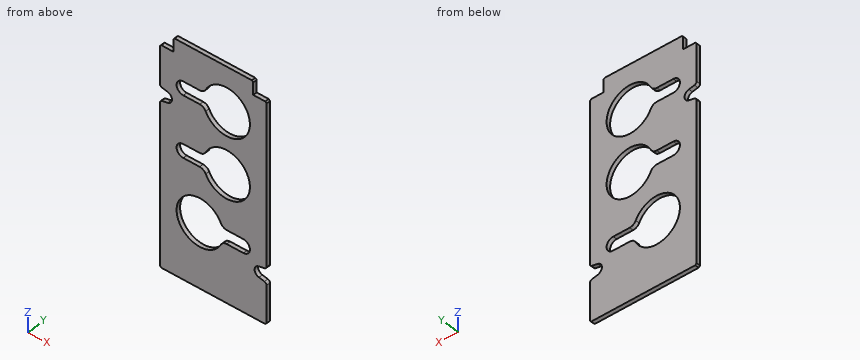
```python
from build123d import *

# Parameters (mm, degrees)
SKETCH226_R     = 17.5
PAD114_DEPTH    = 3
POCKET054_DEPTH = 3.001
FILLET072_R     = 2
CHAMFER079_SIZE = 1
POCKET055_DEPTH = 5
FILLET073_R     = 5


with BuildPart() as part:
    # Sketch226 → Pad114 (new body)
    with BuildSketch(Plane.XZ):
        Polygon((40, 150), (-40, 150), (-40, 310), (-30, 310), (-30, 320), (30, 320), (30, 310), (40, 310), align=None)
        with Locations((10, 287.5)):
            Circle(SKETCH226_R, mode=Mode.SUBTRACT)
        with Locations((10, 242.5)):
            Circle(SKETCH226_R, mode=Mode.SUBTRACT)
        with Locations((-10, 197.5)):
            Circle(SKETCH226_R, mode=Mode.SUBTRACT)
    extrude(amount=-PAD114_DEPTH)

    # Sketch227 → Pocket054 (cut, through all)
    with BuildSketch(Plane.XZ):
        with BuildLine():
            ThreePointArc((-39, 279.898979), (-45, 275), (-39, 270.101021))
            Line((-39, 270.101021), (-34.2, 271.080816))
            ThreePointArc((-34.2, 271.080816), (-31, 275), (-34.2, 278.919184))
            Line((-34.2, 278.919184), (-39, 279.898979))
        make_face()
        with BuildLine():
            ThreePointArc((39, 180.101021), (45, 185), (39, 189.898979))
            Line((39, 189.898979), (34.2, 188.919184))
            ThreePointArc((34.2, 188.919184), (31, 185), (34.2, 181.080816))
            Line((34.2, 181.080816), (39, 180.101021))
        make_face()
    extrude(amount=-POCKET054_DEPTH, mode=Mode.SUBTRACT)

    # Fillet072
    fillet072_edges = [part.edges().sort_by_distance(p)[0] for p in [
        (40, 1.5, 180),
        (40, 1.5, 190),
        (-40, 1.5, 270),
        (-40, 1.5, 280),
    ]]
    fillet(fillet072_edges, radius=FILLET072_R)

    # Chamfer079
    chamfer079_edges = [part.edges().sort_by_distance(p)[0] for p in [
        (-30, 1.5, 320),
        (-40, 1.5, 310),
        (30, 1.5, 320),
        (40, 1.5, 310),
        (-40, 1.5, 150),
        (40, 1.5, 150),
    ]]
    chamfer(chamfer079_edges, length=CHAMFER079_SIZE)

    # Sketch228 → Pocket055 (cut)
    with BuildSketch(Plane.XZ):
        with BuildLine():
            ThreePointArc((10, 282.5), (15, 287.5), (10, 292.5))
            Line((10, 292.5), (-22.5, 292.5))
            ThreePointArc((-22.5, 292.5), (-27.5, 287.5), (-22.5, 282.5))
            Line((-22.5, 282.5), (10, 282.5))
        make_face()
        with BuildLine():
            ThreePointArc((10, 237.5), (15, 242.5), (10, 247.5))
            Line((10, 247.5), (-22.5, 247.5))
            ThreePointArc((-22.5, 247.5), (-27.5, 242.5), (-22.5, 237.5))
            Line((-22.5, 237.5), (10, 237.5))
        make_face()
        with BuildLine():
            ThreePointArc((-10, 202.5), (-15, 197.5), (-10, 192.5))
            Line((-10, 192.5), (22.5, 192.5))
            ThreePointArc((22.5, 192.5), (27.5, 197.5), (22.5, 202.5))
            Line((22.5, 202.5), (-10, 202.5))
        make_face()
    extrude(amount=-POCKET055_DEPTH, mode=Mode.SUBTRACT)

    # Fillet073
    fillet073_edges = [part.edges().sort_by_distance(p)[0] for p in [
        (-6.77051, 1.5, 292.5),
        (-6.77051, 1.5, 282.5),
        (-6.77051, 1.5, 237.5),
        (-6.77051, 1.5, 247.5),
        (6.77051, 1.5, 192.5),
        (6.77051, 1.5, 202.5),
    ]]
    fillet(fillet073_edges, radius=FILLET073_R)


with BuildPart() as part_1:
    # Body098 placement: moved
    add(part.part.moved(Location((0, 75, 0))))


solid = part_1.part
```
Verification items for the finished model (mm, model axes). Give positions to 0.01 mm unless a question says otherwise; leave off trailing zeros. Order: outer loops, then holes, each group sorted by start corner. A loop starts at its lowest first (then second) coordinate and runs counter-clockwise, first axis right, second up. Notation, with made-up numbers: (19, 9.5) -> (61, 9.5) arc R11 ccw to (61, 21.5) -> close; hole circle Ø1 at (12, 77). An arc over 180 degrees is marked (long way). One line per item, written item: value.
(1) Scan lines: line 1 along Z through (x, y) = (-10, 76.2); line 2 along Z through (x, y) = (10, 76.35); line 3 along X through (y, z) = (77.15, 242.5). Record each from-to range of solid material in increasing order. Write a range as [from, to].
Final values:
line 1: [150, 180], [215, 237.5], [247.5, 282.5], [292.5, 320]
line 2: [150, 192.5], [202.5, 225], [260, 270], [305, 320]
line 3: [-40, -27.5], [27.5, 40]
(2) Gauge pin test, flat ends, axial feed: pin 1 (0.9 mm diameter, centred on x = -34, y = 76.5, fed in from +Z); pin 2 (0.9 mm diameter, centred on y = 76.5, z = 312.5, fed in from +X). Record the tip position at first contact, or that the pin passes through.
Final values:
pin 1: z = 310
pin 2: x = 30
(3) Sectioned sample at A-A on z = 197.5. Record the cut outline in (x, y), then the cut area to 3 significant figures.
Final values:
outline: (-40, 75) -> (-27.5, 75) -> (-27.5, 78) -> (-40, 78) -> close; (27.5, 75) -> (40, 75) -> (40, 78) -> (27.5, 78) -> close
area: 75.0 mm^2
(4) Sectioned sample at C-C on y = 76.45. Count the separate pieces of the cut face and the enclosed holes in it, then the cut area to 3 significant figures.
Final values:
separate pieces: 1
enclosed holes: 3
area: 9,780 mm^2
(5) Sectioned sample at B-B on x = 3. Record the cut outline in (y, z).
Final values:
outline: (75, 150) -> (78, 150) -> (78, 185.78) -> (75, 185.78) -> close; (75, 209.22) -> (78, 209.22) -> (78, 226.46) -> (75, 226.46) -> close; (75, 258.54) -> (78, 258.54) -> (78, 271.46) -> (75, 271.46) -> close; (75, 303.54) -> (78, 303.54) -> (78, 320) -> (75, 320) -> close
